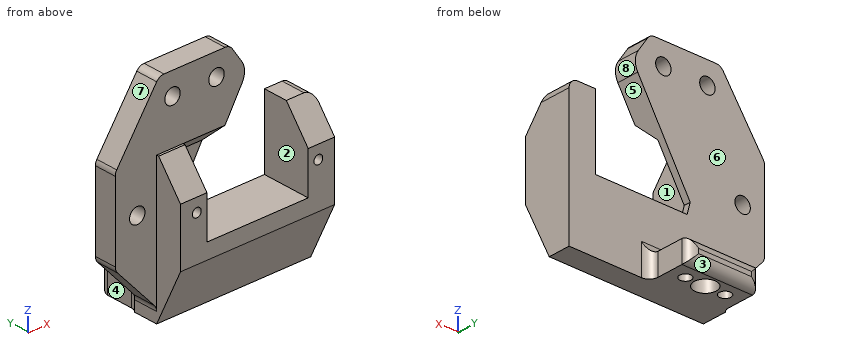
from build123d import *

# Parameters (mm, degrees)
SKETCH1_R                = 1.75
SKETCH1_W                = 7.2
SKETCH1_H                = 5.4
BOSS_EXTRUDE1_DEPTH      = 5
FILLET5_RADIUS           = 10
FILLET5_LENGTH           = 5
FILLET2_R                = 5.4
FILLET6_R                = 5.4
SKETCH3_W                = 35
SKETCH3_H                = 20
SKETCH3_W_2              = 23
SKETCH3_H_2              = 13
BOSS_EXTRUDE4_DEPTH      = 6
SKETCH5_W                = 23
SKETCH5_H                = 13
CUT_EXTRUDE1_DEPTH       = 3.5
CUT_EXTRUDE2_DEPTH       = 76.239617224
SKETCH9_R                = 1
CUT_EXTRUDE4_DEPTH       = 7
BOSS_EXTRUDE5_DEPTH      = 2.5
BOSS_EXTRUDE5_DEPTH_BACK = 2.5
SKETCH10_W               = 16
SKETCH10_H               = 15
SKETCH11_R               = 2.5
SKETCH11_R_2             = 1.3
CUT_EXTRUDE5_DEPTH       = 64.2661837
FILLET8_R                = 2
BOSS_EXTRUDE10_DEPTH     = 35
SKETCH13_W               = 23
SKETCH13_H               = 9.5
CUT_EXTRUDE6_DEPTH       = 3.5
CUT_EXTRUDE7_REACH       = 68.728
BOSS_EXTRUDE11_DEPTH     = 20.6
FILLET9_R                = 2
FILLET10_R               = 2
CUT_EXTRUDE9_DEPTH       = 67.029236021
CUT_EXTRUDE9_DEPTH_BACK  = 67.029236021
FILLET11_R               = 4
CHAMFER1_SIZE            = 3
CHAMFER1_SIZE2           = 2.196152423


# Read off the part's stored shape, not the designer's step: Boss-Extrude11
with BuildPart() as part:
    # Sketch1 → Boss-Extrude1 (new body)
    # profile 1 of 4: a face of its own
    with BuildSketch(Plane(origin=(0, 0, 0), x_dir=(1, 0, 0), z_dir=(0, 1, 0))):
        with BuildLine():
            Line((3.25, 25), (0, 25))
            Line((0, 25), (0, 15))
            Line((0, 15), (10, 0))
            Line((10, 0), (26, 0))
            Line((26, 0), (36, 15))
            Line((36, 15), (60, 15))
            Line((60, 15), (60, 25))
            Line((60, 25), (44.5, 25))
            Line((44.5, 25), (44.5, 19.6))
            Line((44.5, 19.6), (37.3, 19.6))
            Line((37.3, 19.6), (26.5, 19.6))
            Line((26.5, 19.6), (26.5, 25))
            Line((26.5, 25), (6.75, 25))
            ThreePointArc((6.75, 25), (5, 23.25), (3.25, 25))
        make_face()
        with Locations(Location((13, 5, 0), (0, 0, 270))):
            Circle(SKETCH1_R, mode=Mode.SUBTRACT)
        with Locations(Location((23, 5, 0), (0, 0, 270))):
            Circle(SKETCH1_R, mode=Mode.SUBTRACT)
    # profile 2 of 4: a face of its own
    with BuildSketch(Plane(origin=(0, 0, 0), x_dir=(1, 0, 0), z_dir=(0, 1, 0))):
        with BuildLine():
            Line((10, 45), (0, 33.819660113))
            Line((0, 33.819660113), (0, 25))
            Line((0, 25), (3.25, 25))
            ThreePointArc((3.25, 25), (5, 26.75), (6.75, 25))
            Line((6.75, 25), (26.5, 25))
            Line((26.5, 25), (26.5, 30.4))
            Line((26.5, 30.4), (37.3, 30.4))
            Line((37.3, 30.4), (44.5, 30.4))
            Line((44.5, 30.4), (44.5, 25))
            Line((44.5, 25), (60, 25))
            Line((60, 25), (60, 35))
            Line((60, 35), (36, 35))
            Line((36, 35), (26, 45))
            Line((26, 45), (10, 45))
        make_face()
    # profile 3 of 4: a face of its own
    with BuildSketch(Plane(origin=(0, 0, 0), x_dir=(1, 0, 0), z_dir=(0, 1, 0))):
        with Locations((40.9, 27.7)):
            Rectangle(SKETCH1_W, SKETCH1_H)
    # profile 4 of 4: a face of its own
    with BuildSketch(Plane(origin=(0, 0, 0), x_dir=(1, 0, 0), z_dir=(0, 1, 0))):
        with Locations((40.9, 22.3)):
            Rectangle(SKETCH1_W, SKETCH1_H)
    extrude(amount=BOSS_EXTRUDE1_DEPTH)

    # Fillet5: full round fillet: the end face becomes a half cylinder, R = half its width
    fillet5_face = Plane((60, 2.5, -25), x_dir=(0, -1, 0), z_dir=(1, 0, 0))  # on the end face: x along it, z out of the body
    fillet5_slab = fillet5_face.offset(-FILLET5_RADIUS / 2) * Box(FILLET5_LENGTH, 2 * FILLET5_RADIUS, FILLET5_RADIUS, mode=Mode.PRIVATE)  # the body's end, R deep
    fillet5_round = Plane((50, 2.5, -25), x_dir=(1, 0, 0), z_dir=(0, -1, 0)) * Cylinder(FILLET5_RADIUS, FILLET5_LENGTH, mode=Mode.PRIVATE)  # its axis R under the face
    add(fillet5_slab - fillet5_round, mode=Mode.SUBTRACT)

    # Fillet2
    fillet2_edges = [part.edges().sort_by_distance(p)[0] for p in [
        (26.5, 2.5, -30.4),
        (26.5, 2.5, -19.6),
    ]]
    fillet(fillet2_edges, radius=FILLET2_R - 0.0001)  # a hair under: the kernel refuses the full size

    # Fillet6
    fillet6_edges = [part.edges().sort_by_distance(p)[0] for p in [
        (37.3, 2.5, -19.6),
        (37.3, 2.5, -30.4),
    ]]
    fillet(fillet6_edges, radius=FILLET6_R - 0.0001)  # a hair under: the kernel refuses the full size

    # Sketch3 → Boss-Extrude4 (add)
    with BuildSketch(Plane.XZ):
        with Locations((26.9, -25)):
            Rectangle(SKETCH3_W, SKETCH3_H)
        with Locations((26.9, -25)):
            Rectangle(SKETCH3_W_2, SKETCH3_H_2, mode=Mode.SUBTRACT)
    extrude(amount=BOSS_EXTRUDE4_DEPTH)

    # Sketch5 → Cut-Extrude1 (cut)
    with BuildSketch(Plane.XZ):
        with Locations((26.9, -25)):
            Rectangle(SKETCH5_W, SKETCH5_H)
    extrude(amount=-CUT_EXTRUDE1_DEPTH, mode=Mode.SUBTRACT)

    # Sketch6 → Cut-Extrude2 (cut, through all)
    with BuildSketch(Plane.XZ):
        with BuildLine():
            Line((44.4, -15), (44.4, -35))
            Line((44.4, -35), (50, -35))
            ThreePointArc((50, -35), (60, -25), (50, -15))
            Line((50, -15), (44.4, -15))
        make_face()
    extrude(amount=-CUT_EXTRUDE2_DEPTH, mode=Mode.SUBTRACT)

    # Sketch9 → Cut-Extrude4 (cut)
    with BuildSketch(Plane.XZ.offset(6)):
        with Locations(Location((13.1, -25, 0), (0, 0, 270))):
            Circle(SKETCH9_R)
        with Locations(Location((40.7, -25, 0), (0, 0, 270))):
            Circle(SKETCH9_R)
    extrude(amount=-CUT_EXTRUDE4_DEPTH, mode=Mode.SUBTRACT)

    # Sketch10 → Boss-Extrude5 (add, two sides: drawn at the far end of the back side and taken through both)
    with BuildSketch(Plane(origin=(0, 0, -45), x_dir=(-1, 0, 0), z_dir=(0, 0, -1)).offset(-BOSS_EXTRUDE5_DEPTH_BACK)):
        with Locations((-18, 7.5)):
            Rectangle(SKETCH10_W, SKETCH10_H)
    extrude(amount=BOSS_EXTRUDE5_DEPTH + BOSS_EXTRUDE5_DEPTH_BACK)

    # Sketch11 → Cut-Extrude5 (cut, through all)
    with BuildSketch(Plane.XY.offset(-42.5)):
        with Locations((18, 10)):
            Circle(SKETCH11_R)
        with Locations((22.5, 10)):
            Circle(SKETCH11_R_2)
        with Locations((13.5, 10)):
            Circle(SKETCH11_R_2)
    extrude(amount=-CUT_EXTRUDE5_DEPTH, mode=Mode.SUBTRACT)

    # Fillet8
    fillet8_edges = [part.edges().sort_by_distance(p)[0] for p in [
        (26, 15, -45),
        (18, 15, -42.5),
        (10, 15, -45),
        (18, 15, -47.5),
    ]]
    fillet(fillet8_edges, radius=FILLET8_R)

    # Sketch12 → Boss-Extrude10 (add)
    with BuildSketch(Plane(origin=(44.4, 0, 0), x_dir=(0, 0, -1), z_dir=(1, 0, 0))):
        Polygon((35, -6), (35, 5), (47.5, 5), (47.5, 0), align=None)
    extrude(amount=-BOSS_EXTRUDE10_DEPTH)

    # Sketch13 → Cut-Extrude6 (cut)
    with BuildSketch(Plane(origin=(0, 0, -18.5), x_dir=(-1, 0, 0), z_dir=(0, 0, -1))):
        with Locations((-26.9, -1.25)):
            Rectangle(SKETCH13_W, SKETCH13_H)
    extrude(amount=-CUT_EXTRUDE6_DEPTH, mode=Mode.SUBTRACT)

    # Cut-Extrude7: up to this face of the body (flat: up to its plane)
    cut_extrude7_end = Plane(part.part.faces().sort_by_distance((9.4, -2.280677184, -29.977280777))[0])
    # Sketch14 → Cut-Extrude7 (cut, up to the picked face)
    with BuildSketch(Plane(origin=(44.4, 0, 0), x_dir=(0, 0, -1), z_dir=(1, 0, 0)), mode=Mode.PRIVATE) as cut_extrude7_sk1:
        Polygon((15, -0.5), (22, -6), (15, -6), align=None)
    cut_extrude7_tool1 = split(extrude(cut_extrude7_sk1.sketch, amount=-CUT_EXTRUDE7_REACH, mode=Mode.PRIVATE), bisect_by=cut_extrude7_end, keep=Keep.BOTH, mode=Mode.PRIVATE)
    add(cut_extrude7_tool1.solids().sort_by(Axis((44.4, -4.166667, -17.333333), (-1, 0, 0)))[0], mode=Mode.SUBTRACT)

    # Boss-Extrude11 outline → Boss-Extrude11 (add)
    with BuildSketch(Plane(origin=(15.4, 0, 0), x_dir=(0, 0, -1), z_dir=(1, 0, 0))):
        Polygon((15, 0), (18.5, 3.5), (15, 3.5), align=None)
    extrude(amount=BOSS_EXTRUDE11_DEPTH)

    # Fillet9
    fillet9_edges = [part.edges().sort_by_distance(p)[0] for p in [
        (9.4, 2.5, -44.329179607),
        (44.4, 2.25, -15),
        (36, 4.25, -15),
        (26, 2.5, 0),
        (10, 2.5, 0),
        (0, 2.5, -15),
        (0, 2.5, -33.819660113),
    ]]
    fillet(fillet9_edges, radius=FILLET9_R)

    # Fillet10
    fillet10_edges = [part.edges().sort_by_distance(p)[0] for p in [
        (10, 5, -45),
        (26, 5, -45),
        (18, 5, -42.5),
    ]]
    fillet(fillet10_edges, radius=FILLET10_R)

    # Sketch18 → Cut-Extrude9 (cut, two sides: drawn at the far end of the back side and taken through both)
    with BuildSketch(Plane.XZ.offset(-3.5).offset(-CUT_EXTRUDE9_DEPTH_BACK)):
        Polygon((15.4, -31.5), (38.4, -31.5), (38.4, 8.337168574), align=None)
    extrude(amount=CUT_EXTRUDE9_DEPTH + CUT_EXTRUDE9_DEPTH_BACK, mode=Mode.SUBTRACT)

    # Fillet11
    fillet11_edges = [part.edges().sort_by_distance(p)[0] for p in [
        (30.065611038, 2.5, -6.098416558),
    ]]
    fillet(fillet11_edges, radius=FILLET11_R)

    # Chamfer1
    chamfer1_edges = [part.edges().sort_by_distance(p)[0] for p in [
        (15.4, 4.25, -31.5),
    ]]
    chamfer1_side = [part.faces().sort_by_distance(p)[0] for p in [
        (24.055872114, 3.154417612, -16.507589715),
    ]]
    chamfer(chamfer1_edges, length=CHAMFER1_SIZE, length2=CHAMFER1_SIZE2, reference=chamfer1_side[0])


solid = part.part
Source: CAD feature listing. Evaluate the final solid. Frame: model axes, mm. Face numbers are marked on the shaded views. A direction names the side the tool comes from. Coordinates: 2 decimals unless noted, no trailing zeros. Loops run counter-clockwise (first coordinate to the right, second up) from the corner with the lowest first, then second, coordinate; pieces in that order, holes last. Notation, with made-up numbers: (84, 22) - (88, 22) arc R22 ccw to (88, 34) - close; hole circle Ø3 at (69.5, 60). An arc over 180 degrees is marked (long way). Return JSON: item names as keys, results as strings.
Q1. Section D-D, the plane z = -5. Return loops of the section in (x, y).
Results:
{"outline": "(6.67, 0) - (11.25, 0) - (11.25, 5) - (6.67, 5) - close; (14.75, 0) - (21.25, 0) - (21.25, 5) - (14.75, 5) - close; (24.75, 0) - (29.16, 0) - (29.16, 5) - (24.75, 5) - close"}
Q2. Material intervals for line 1 along X through (y, z) = (-3.25, -25); line 2 along Y through (x, z) = (4, -34.5); line 3 along Y through (x, z) = (37, -34), sorted ascending.
Results:
{"line 1": "9.4 to 12.1, 14.1 to 15.4, 38.4 to 39.7, 41.7 to 44.4", "line 2": "0 to 5", "line 3": "-6 to 5"}
Q3. Access query for the marked faces 1, 2, 3, 4 and 5. Directions: +Z, -Z, +X, -X, +Y, -Y. A direction counts if a zero-diameter tool reaches every point of the face in a straight line with its end or side. Return the directions, or none.
Results:
{"face 1": "-Y", "face 2": "+Z, +Y, -Y", "face 3": "-Z, +X, -X, +Y", "face 4": "+Z, -Z, -X, +Y", "face 5": "+Y, -Y"}
Q4. Section A-A, the plane z = -25. Return loops of the section in (x, y), plus the area to 3 significant figures.
Results:
{"outline": "(0, 0) - (3.25, 0) - (3.25, 5) - (0, 5) - close; (6.75, 0) - (9.4, 0) - (9.4, -6) - (12.1, -6) - (12.1, 1) - (14.1, 1) - (14.1, -6) - (15.4, -6) - (15.4, 3.5) - (19.15, 3.5) - (19.15, 5) - (6.75, 5) - close; (38.4, -6) - (39.7, -6) - (39.7, 1) - (41.7, 1) - (41.7, -6) - (44.4, -6) - (44.4, 5) - (38.4, 5) - close", "area": "139 mm2"}
Q5. Section C-C, the plane y = 2. Return loops of the section in (x, z).
Results:
{"outline": "(0, -33.06) arc R2 ccw to (0.51, -34.39) - (8.89, -43.76) arc R2 cw to (9.4, -45.09) - (9.4, -47.5) - (44.4, -47.5) - (44.4, -17) arc R2 ccw to (42.4, -15) - (38.4, -15) - (38.4, -31.5) - (15.4, -31.5) - (15.4, -17) - (23.77, -17) - (28.82, -8.25) arc R4 ccw to (28.69, -4.03) - (26.59, -0.89) arc R2 ccw to (24.93, 0) - (11.07, 0) arc R2 ccw to (9.41, -0.89) - (0.34, -14.5) arc R2 ccw to (0, -15.61) - close; hole circle Ø3.5 at (5, -25); hole circle Ø3.5 at (13, -5); hole circle Ø3.5 at (23, -5)"}
Q6. Mould query, pull axis Z, two halves, no side actions, for the marked faces 6, 7 and 8. Classes: released by +Z, released by -Z, zero draft, split by the parting line, or undercut.
Results:
{"face 6": "zero draft", "face 7": "released by +Z", "face 8": "undercut"}
Q7. Contact query for flat-ended pins moving along their axis: P1, Ø2.5, axis at y = 9, z = -46, coming from the +X side; P2, Ø3, axis at x = 27, z = -10.5, coming from the +Y side; P3, Ø10, axis at x = 32.5, y = 7.5, coming from the -Z side; P4, Ø5.5, axis at x = 5, z = -25, coming from the -Y side. Output: stop coordinate, or through.
Results:
{"P1": "x = 26", "P2": "y = 5", "P3": "z = -47.5", "P4": "y = 0"}
Q8. Section B-B, the plane x = 5. Return loops of the section in (y, z).
Results:
{"outline": "(0, -39.41) - (5, -39.41) - (5, -26.75) - (0, -26.75) - close; (0, -23.25) - (5, -23.25) - (5, -7.5) - (0, -7.5) - close"}
